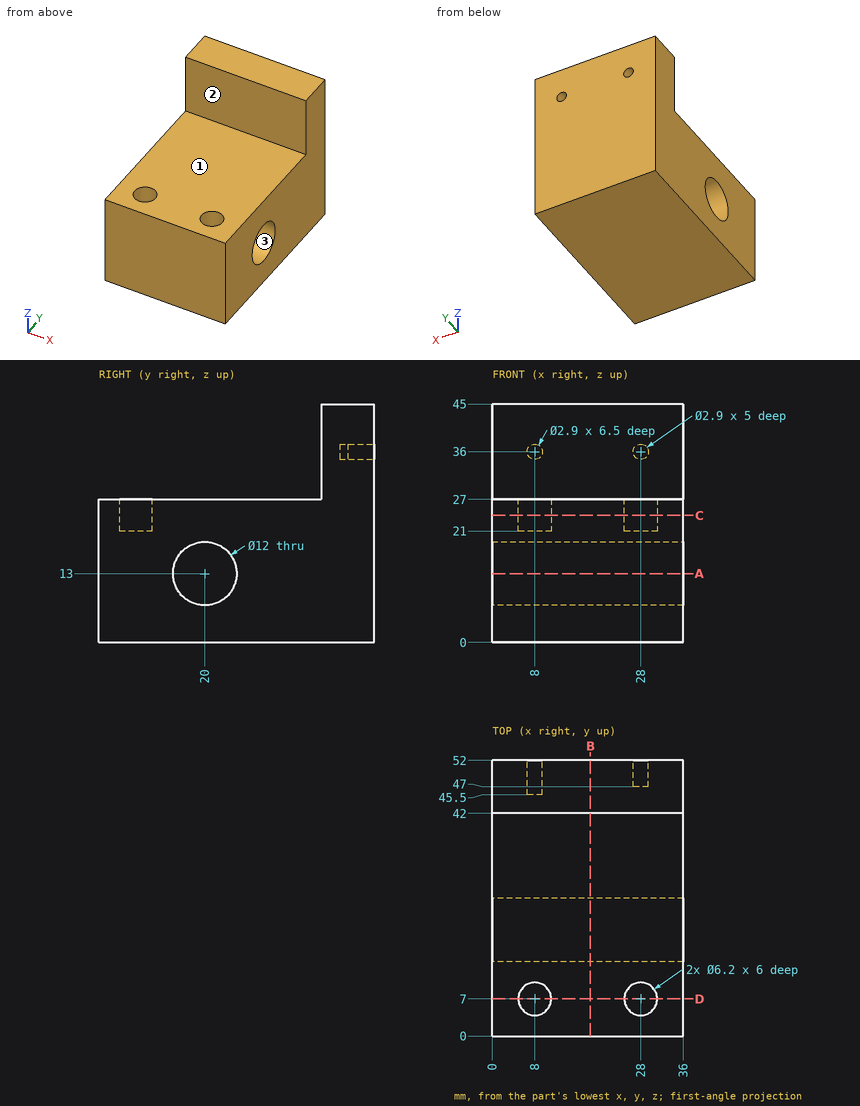
Verification items for this drawing (mm, ordinates from the low corner). Give positions to 0.01 mm unless a question says otherwise; leave off trailing zeros. Loops run counter-clockwise (first coordinate to the right, second up) from the corner with the lowest first, then second, coordinate; pieces in that order, holes last.
(1) Release check for a two-part mould opening along Y. For the marked faces 1, 2 and 3 record: released by +Y, released by -Y, zero draft, split by the parting line, or undercut.
From the geometry:
face 1: zero draft
face 2: released by -Y
face 3: undercut
(2) Section check D-D on y = 7. Record the cut outline in (x, z).
From the geometry:
outline: (0, 0) - (36, 0) - (36, 27) - (31.1, 27) - (31.1, 21) - (24.9, 21) - (24.9, 27) - (11.1, 27) - (11.1, 21) - (4.9, 21) - (4.9, 27) - (0, 27) - close
(3) Section check B-B on x = 18.5. Record the cut outline in (y, z).
From the geometry:
outline: (0, 0) - (52, 0) - (52, 45) - (42, 45) - (42, 27) - (0, 27) - close; hole circle Ø12 at (20, 13)
(4) Depth check by flat-ended pin: pin 1 Ø4 at (x, z) = (8, 36) entering from -Y; pin 2 Ø7 at (x, y) = (9, 6) entering from +Z; pin 3 Ø12 at (y, z) = (26, 37.5) entering from +X; pin 4 Ø5 at (x, y) = (8, 7) entering from +Z. Enter the tip coordinate at first touch or a pass-through.
From the geometry:
pin 1: stops at y = 42
pin 2: stops at z = 27
pin 3: passes through
pin 4: stops at z = 21
(5) Thickness scan on L1, parallel to X at y = 50, z = 36; L2, parallel to Y at x = 15, z = 13; L3, parallel to Y at x = 8, z = 23. Record the ranges inside material, lowest first.
From the geometry:
L1: x = 0 to 6.55, 9.45 to 26.55, 29.45 to 36
L2: y = 0 to 14, 26 to 52
L3: y = 0 to 3.9, 10.1 to 52
(6) Section check C-C on z = 24. Record the cut outline in (x, y).
From the geometry:
outline: (0, 0) - (36, 0) - (36, 52) - (0, 52) - close; hole circle Ø6.2 at (8, 7); hole circle Ø6.2 at (28, 7)
(7) Section check A-A on z = 13. Record the cut outline in (x, y).
From the geometry:
outline: (0, 0) - (36, 0) - (36, 14) - (0, 14) - close; (0, 26) - (36, 26) - (36, 52) - (0, 52) - close
